from build123d import *

# Parameters (mm, degrees)
SKETCH_2_R      = 2.05
SKETCH_2_R_2    = 44.910539349
EXTRUDE_1_DEPTH = 1


with BuildPart() as part:
    # 草图1 → 旋转1 (revolve)
    with BuildSketch(Plane.XY):
        with BuildLine():
            ThreePointArc((-45.813874016, -0.428936451), (-43.539426354, -2.86488143), (-40.275857757, -3.540203663))
            ThreePointArc((-40.275857757, -3.540203663), (-35.905809817, -1.000028754), (-31.553091654, -3.569785971))
            Line((-31.553091654, -3.569785971), (-27, -3.569785971))
            Line((-27, -3.569785971), (-27, -2.569785971))
            Line((-27, -2.569785971), (-31, -2.569785971))
            ThreePointArc((-31, -2.569785971), (-35.922766673, 0), (-40.845533346, -2.569785971))
            ThreePointArc((-40.845533346, -2.569785971), (-43.250116145, -1.873465974), (-44.910539349, 0))
            Line((-44.910539349, 0), (-45.813874016, -0.428936451))
        make_face()
    revolve(axis=Axis((0, 6.917160425, 0), (0, -1, 0)))

    # 草图2 → 凸台-拉伸1 (add)
    with BuildSketch(Plane(origin=(0, 0, 0), x_dir=(1, 0, 0), z_dir=(0, 1, 0))):
        with BuildLine():
            Line((43.25, 47.25), (-43.25, 47.25))
            ThreePointArc((-43.25, 47.25), (-46.078427125, 46.078427125), (-47.25, 43.25))
            Line((-47.25, 43.25), (-47.25, -43.25))
            ThreePointArc((-47.25, -43.25), (-46.078427125, -46.078427125), (-43.25, -47.25))
            Line((-43.25, -47.25), (43.25, -47.25))
            ThreePointArc((43.25, -47.25), (46.078427125, -46.078427125), (47.25, -43.25))
            Line((47.25, -43.25), (47.25, 43.25))
            ThreePointArc((47.25, 43.25), (46.078427125, 46.078427125), (43.25, 47.25))
        make_face()
        with Locations((-40.658639918, -40.658639918)):
            Circle(SKETCH_2_R, mode=Mode.SUBTRACT)
        with Locations((40.658639918, -40.658639918)):
            Circle(SKETCH_2_R, mode=Mode.SUBTRACT)
        with Locations((-40.658639918, 40.658639918)):
            Circle(SKETCH_2_R, mode=Mode.SUBTRACT)
        Circle(SKETCH_2_R_2, mode=Mode.SUBTRACT)
        with Locations((40.658639918, 40.658639918)):
            Circle(SKETCH_2_R, mode=Mode.SUBTRACT)
    extrude(amount=-EXTRUDE_1_DEPTH)


solid = part.part
Can you work these out from the model? Positions are in its coordinate system, mm. A direction names the side the tool comes from. Round coordinates to 2 decimals unless told otherwise and drop trailing zeros. Loops run counter-clockwise (first coordinate to the right, second up) from the corner with the lowest first, then second, coordinate; pieces in that order, holes last. Notation, with made-up numbers: (-29.75, 52.5) - (9.25, 52.5) arc R13 ccw to (9.25, 64.5) - close; hole circle Ø1 at (-38, 17.5). An arc over 180 degrees is marked (long way). Answer in a Markdown table with one row per item. Add a question column.
Q1. I want a section at A-A on y = -1.85. List the corners of the cut face in (x, z) for me.
Q2. For pin 1 Ø4 at (x, z) = (-21.5, -35) entering from +Y; pin 2 Ø1 at (y, z) = (-3, -14.5) entering from -X; pin 3 Ø3.5 at (x, z) = (-40.66, -40.66) entering from -Y; pin 4 Ø5.5 at (x, z) = (40.66, 40.66) entering from -Y, each with a flat end and sliding along its axis, tell me the tip position at first contact or that it passes through.
Q3. I need wall thicknesses on L1, parallel to Z at x = 8, y = -0.8; L2, parallel to Z at x = -22.5, y = -3; L3, parallel to X at y = -2.7, z = 10.5. Which ranges of each line are inside material? Lowest first, please.
Q4. Which directions (+Z, -Z, +X, -X, +Y, -Y) give clear straight access to the entire face, cutting with the end or side of a thin tool? Please do faces 5 (the flat face through (-25, -1, -39)), 6 (the flat face through (2, -2.57, -28)), 7 (the cylindrical face through (-42.17, -0.493, -42.044)).
Q5. I want a section at C-C on z = 0. List the corners of the cut face in (x, y) for me.
Q6. I want a section at B-B on x = 0. List the corners of the cut face in (y, z) for me, and give its area (3 significant figures).
Q7. We'd pull the mould along Z, two halves only. Please class faces 1 (the flat face through (-23.2, -3.57, -14.2)), 2 (the cylindrical face through (46.109, -0.493, -46.047)), 3 (the cylindrical face through (-42.707, -0.493, 40.569)), 4 (the cylindrical face through (-46.109, -0.493, 46.047)): pulls with the +Z half, pulls with the -Z half, needs draft (parallel to the pull), parting line crosses it, or undercut.
A:
| question | item | result |
|---|---|---|
| 1 | outline | circle Ø89.68 at (0, 0); circle Ø80.51 at (0, 0); circle Ø66.27 at (0, 0); hole circle Ø86.57 at (0, 0); hole circle Ø77.42 at (0, 0); hole circle Ø63.18 at (0, 0) |
| 2 | pin 1 | y = -0.9 |
| 2 | pin 2 | x = -41.67 |
| 2 | pin 3 | through |
| 2 | pin 4 | y = -1 |
| 3 | L1 | -47.25 to -43.7, -38.08 to -31.94, 31.94 to 38.08, 43.7 to 47.25 |
| 3 | L2 | -36.98 to -32.98, -22.65 to -14.92, 14.92 to 22.65, 32.98 to 36.98 |
| 3 | L3 | -42.54 to -38.26, -30.4 to -24.87, 24.87 to 30.4, 38.26 to 42.54 |
| 4 | face 5 | -Y |
| 4 | face 6 | +Y |
| 4 | face 7 | +Y, -Y |
| 5 | outline | (-47.25, -1) - (-45.5, -1) arc R5.5 ccw to (-40.28, -3.54) arc R5 cw to (-31.55, -3.57) - (-27, -3.57) - (-27, -2.57) - (-31, -2.57) arc R6 ccw to (-40.85, -2.57) arc R4.5 cw to (-44.91, 0) - (-47.25, 0) - close; (27, -3.57) - (31.55, -3.57) arc R5 cw to (40.28, -3.54) arc R5.5 ccw to (45.5, -1) - (47.25, -1) - (47.25, 0) - (44.91, 0) arc R4.5 cw to (40.85, -2.57) arc R6 ccw to (31, -2.57) - (27, -2.57) - close |
| 6 | outline | (-3.57, -31.55) arc R5 cw to (-3.54, -40.28) arc R5.5 ccw to (-1, -45.5) - (-1, -47.25) - (0, -47.25) - (0, -44.91) arc R4.5 cw to (-2.57, -40.85) arc R6 ccw to (-2.57, -31) - (-2.57, -27) - (-3.57, -27) - close; (-3.57, 27) - (-2.57, 27) - (-2.57, 31) arc R6 ccw to (-2.57, 40.85) arc R4.5 cw to (0, 44.91) - (0, 47.25) - (-1, 47.25) - (-1, 45.5) arc R5.5 ccw to (-3.54, 40.28) arc R5 cw to (-3.57, 31.55) - close |
| 6 | area | 46.0 mm^2 |
| 7 | face 1 | needs draft |
| 7 | face 2 | pulls with the -Z half |
| 7 | face 3 | undercut |
| 7 | face 4 | pulls with the +Z half |
